Model file for the job. Use its own axes, mm. Face numbers are marked on the shaded views. A direction names the side the tool comes from. Round coordinates to 2 decimals unless told otherwise and drop trailing zeros. Loops run counter-clockwise (first coordinate to the right, second up) from the corner with the lowest first, then second, coordinate; pieces in that order, holes last. Notation, with made-up numbers: M 3.25,-36 L 54.25,-36 A8 cw 54.25,-28 Z; hole C 3,81.5 d10. An arc over 180 degrees is marked long. Use a Markdown table: item, result. Add a question column.
Q1. Cut at B-B (z = 47.5). Give the cut face in (x, y).
Q2. Probe line 1 (X direction, y = 0, z = 21.5); line 2 (Y direction, x = -13.5, z = 3.5); line 3 (Z direction, x = 4.5, y = 39). List the from-to ranges inside material, lowest first. Write a range as from..to.
Q3. Cut at C-C (x = -13). Give the cut face in (y, z), plus the area to 3 significant figures.
Q4. Tool access for the marked faces 1 and 2: list every direction of +Z, -Z, +X, -X, +Y, -Y with a clear straight run to the whole face (end or side of a thin tool).
Q5. Cut at D-D (y = 11). Give the cut face in (x, z), plus the area to 3 significant figures.
Q6. Mould opens along Y. For the marked faces 3, 4 and 5 say: +Y half, -Y half, draft (parallel to the pull), parting line (faces both ways), or undercut.
Q7. Cut at A-A (y = 34). Give the cut face in (x, z).
Q8. Pin check, flat tip, straight feed: pin 1 (4 mm diameter, centred on x = 1.5, y = -9.5, fed in from +Z). Stop position of the tip, or through.
from build123d import *
from build123d import SkipClean  # not in build123d's __all__

# Parameters (mm, degrees)
F1_DEPTH = 50.8
F2_W     = 31.0465274379
F2_H     = 13.5299048007
F3_DEPTH = 25.4
F5_DEPTH = 25.4


with BuildPart() as f1:
    # F0 (on Top) → F1 (new body)
    with BuildSketch(Plane.XY):
        Polygon((-62.0559491217, 14.3422799075), (-67.1168267727, 14.3422799075), (-67.1168267727, -12.8931785002), (-13.6161604896, -12.8931785002), (-13.6161604896, -7.8323045745), (-62.0559491217, -7.8323045745), align=None)
    extrude(amount=F1_DEPTH)

    # F2 (on face) → F3 (cut)
    with BuildSketch(Plane.XZ.offset(12.8931785002)):
        with Locations((-29.1394242086, 44.0350475997)):
            Rectangle(F2_W, F2_H)
    extrude(amount=-F3_DEPTH, mode=Mode.SUBTRACT)

    # F4 (on face) → F5 (cut)
    with BuildSketch(Plane(origin=(-67.1168267727, 0, 0), x_dir=(0, -1, 0), z_dir=(-1, 0, 0))):
        with BuildLine():
            ThreePointArc((-14.3422799075, 20.8923586581), (-11.1548961475, 22.21261624), (-9.8346385657, 25.4))
            ThreePointArc((-9.8346385657, 25.4), (-11.1548961475, 28.58738376), (-14.3422799075, 29.9076413419))
            Line((-14.3422799075, 29.9076413419), (-14.3422799075, 20.8923586581))
        make_face()
    extrude(amount=-F5_DEPTH, mode=Mode.SUBTRACT)

    # F6: F1 across face


with BuildPart() as f1_1:
    add(f1.part, clean=False)
    with SkipClean():  # cleaning this boolean's faces spoils the solid; the shape is the same uncleaned
        add(f1.part.mirror(Plane(origin=(-64.5863879472, 14.3422799075, 10.4461793291), x_dir=(-1, 0, 0), z_dir=(0, 1, 0))), clean=False)

    # F7: F1 across face


with BuildPart() as f1_2:
    add(f1_1.part, clean=False)
    add(f1_1.part.mirror(Plane(origin=(-13.6161604896, 39.0473013524, 18.6350475997), x_dir=(0, 1, 0), z_dir=(1, 0, 0))), clean=False)


solid = f1_2.part
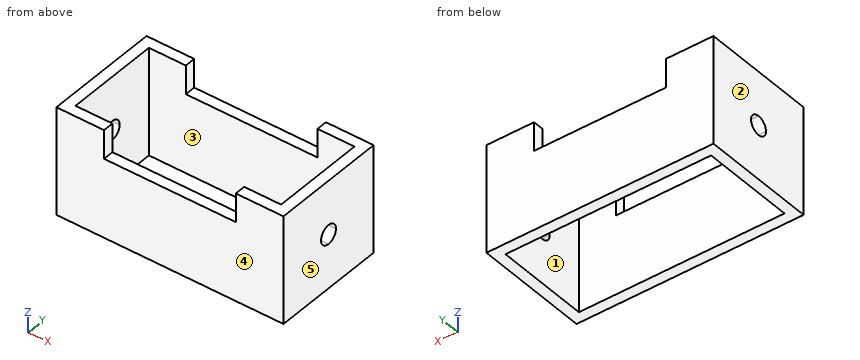
Checked values:
| question | item | result |
|---|---|---|
| 1 | outline | M -67.12,-12.89 L -44.66,-12.89 L -44.66,-7.83 L -62.06,-7.83 L -62.06,36.52 L -44.66,36.52 L -44.66,41.58 L -67.12,41.58 Z; M 17.43,-12.89 L 39.88,-12.89 L 39.88,41.58 L 17.43,41.58 L 17.43,36.52 L 34.82,36.52 L 34.82,-7.83 L 17.43,-7.83 Z |
| 2 | line 1 | x = -67.12..-62.06, 34.82..39.88 |
| 2 | line 2 | y = -12.89..-7.83, 36.52..41.58 |
| 2 | line 3 | z = 0..37.27 |
| 3 | outline | M -12.89,0 L -7.83,0 L -7.83,37.27 L -12.89,37.27 Z; M 36.52,0 L 41.58,0 L 41.58,37.27 L 36.52,37.27 Z |
| 3 | area | 377 mm^2 |
| 4 | face 1 | +Z, -Z |
| 4 | face 2 | +Z, -Z, -X, +Y, -Y |
| 5 | outline | M -67.12,0 L -62.06,0 L -62.06,22.38 L -67.12,22.38 Z; M -67.12,28.42 L -62.06,28.42 L -62.06,50.8 L -67.12,50.8 Z; M 34.82,0 L 39.88,0 L 39.88,22.38 L 34.82,22.38 Z; M 34.82,28.42 L 39.88,28.42 L 39.88,50.8 L 34.82,50.8 Z |
| 5 | area | 453 mm^2 |
| 6 | face 3 | undercut |
| 6 | face 4 | -Y half |
| 6 | face 5 | draft |
| 7 | outline | M -67.12,0 L -62.06,0 L -62.06,50.8 L -67.12,50.8 Z; M 34.82,0 L 39.88,0 L 39.88,50.8 L 34.82,50.8 Z |
| 8 | pin 1 | stops at z = 37.27 |
